```python
from build123d import *

# Parameters (mm, degrees)
F1_DEPTH = 3


with BuildPart() as f1:
    # F0 (on Top) → F1 (new body)
    with BuildSketch(Plane.XY):
        with BuildLine():
            Line((-2, 29.9332590942), (-2, 37.4466286867))
            ThreePointArc((-2, 37.4466286867), (-26.5165042945, 26.5165042945), (-37.4466286867, 2))
            Line((-37.4466286867, 2), (-29.9332590942, 2))
            ThreePointArc((-29.9332590942, 2), (-21.2132034356, 21.2132034356), (-2, 29.9332590942))
        make_face()
        with BuildLine():
            Line((-29.9332590942, -2), (-37.4466286867, -2))
            ThreePointArc((-37.4466286867, -2), (-26.5165042945, -26.5165042945), (-2, -37.4466286867))
            Line((-2, -37.4466286867), (-2, -29.9332590942))
            ThreePointArc((-2, -29.9332590942), (-21.2132034356, -21.2132034356), (-29.9332590942, -2))
        make_face()
        with BuildLine():
            Line((-14.8660687473, -2), (-27.4271763038, -2))
            ThreePointArc((-27.4271763038, -2), (-19.4454364826, -19.4454364826), (-2, -27.4271763038))
            Line((-2, -27.4271763038), (-2, -14.8660687473))
            ThreePointArc((-2, -14.8660687473), (-10.6066017178, -10.6066017178), (-14.8660687473, -2))
        make_face()
        with BuildLine():
            Line((-2, 14.8660687473), (-2, 27.4271763038))
            ThreePointArc((-2, 27.4271763038), (-19.4454364826, 19.4454364826), (-27.4271763038, 2))
            Line((-27.4271763038, 2), (-14.8660687473, 2))
            ThreePointArc((-14.8660687473, 2), (-10.6066017178, 10.6066017178), (-2, 14.8660687473))
        make_face()
        with BuildLine():
            ThreePointArc((27.4271763038, 2), (19.4454364826, 19.4454364826), (2, 27.4271763038))
            Line((2, 27.4271763038), (2, 14.8660687473))
            ThreePointArc((2, 14.8660687473), (10.6066017178, 10.6066017178), (14.8660687473, 2))
            Line((14.8660687473, 2), (27.4271763038, 2))
        make_face()
        with BuildLine():
            ThreePointArc((2, -27.4271763038), (19.4454364826, -19.4454364826), (27.4271763038, -2))
            Line((27.4271763038, -2), (14.8660687473, -2))
            ThreePointArc((14.8660687473, -2), (10.6066017178, -10.6066017178), (2, -14.8660687473))
            Line((2, -14.8660687473), (2, -27.4271763038))
        make_face()
        with BuildLine():
            ThreePointArc((2, -37.4466286867), (26.5165042945, -26.5165042945), (37.4466286867, -2))
            Line((37.4466286867, -2), (29.9332590942, -2))
            ThreePointArc((29.9332590942, -2), (21.2132034356, -21.2132034356), (2, -29.9332590942))
            Line((2, -29.9332590942), (2, -37.4466286867))
        make_face()
        with BuildLine():
            ThreePointArc((37.4466286867, 2), (26.5165042945, 26.5165042945), (2, 37.4466286867))
            Line((2, 37.4466286867), (2, 29.9332590942))
            ThreePointArc((2, 29.9332590942), (21.2132034356, 21.2132034356), (29.9332590942, 2))
            Line((29.9332590942, 2), (37.4466286867, 2))
        make_face()
        with BuildLine():
            Line((2, 14.8660687473), (2, 27.4271763038))
            ThreePointArc((2, 27.4271763038), (0, 27.5), (-2, 27.4271763038))
            Line((-2, 27.4271763038), (-2, 14.8660687473))
            ThreePointArc((-2, 14.8660687473), (0, 15), (2, 14.8660687473))
        make_face()
        with BuildLine():
            Line((2, 27.4271763038), (2, 29.9332590942))
            ThreePointArc((2, 29.9332590942), (0, 30), (-2, 29.9332590942))
            Line((-2, 29.9332590942), (-2, 27.4271763038))
            ThreePointArc((-2, 27.4271763038), (0, 27.5), (2, 27.4271763038))
        make_face()
        with BuildLine():
            Line((2, 29.9332590942), (2, 37.4466286867))
            Line((2, 37.4466286867), (-2, 37.4466286867))
            Line((-2, 37.4466286867), (-2, 29.9332590942))
            ThreePointArc((-2, 29.9332590942), (0, 30), (2, 29.9332590942))
        make_face()
        with BuildLine():
            Line((2, 12.3389626793), (2, 14.8660687473))
            ThreePointArc((2, 14.8660687473), (0, 15), (-2, 14.8660687473))
            Line((-2, 14.8660687473), (-2, 12.3389626793))
            ThreePointArc((-2, 12.3389626793), (0, 12.5), (2, 12.3389626793))
        make_face()
        with BuildLine():
            Line((2, 2.8722813233), (2, 12.3389626793))
            ThreePointArc((2, 12.3389626793), (0, 12.5), (-2, 12.3389626793))
            Line((-2, 12.3389626793), (-2, 2.8722813233))
            ThreePointArc((-2, 2.8722813233), (0, 3.5), (2, 2.8722813233))
        make_face()
        with BuildLine():
            Line((-2.8722813233, 2), (-12.3389626793, 2))
            ThreePointArc((-12.3389626793, 2), (-12.5, 0), (-12.3389626793, -2))
            Line((-12.3389626793, -2), (-2.8722813233, -2))
            ThreePointArc((-2.8722813233, -2), (-3.5, 0), (-2.8722813233, 2))
        make_face()
        with BuildLine():
            Line((-14.8660687473, 2), (-27.4271763038, 2))
            ThreePointArc((-27.4271763038, 2), (-27.5, 0), (-27.4271763038, -2))
            Line((-27.4271763038, -2), (-14.8660687473, -2))
            ThreePointArc((-14.8660687473, -2), (-15, 0), (-14.8660687473, 2))
        make_face()
        with BuildLine():
            Line((-12.3389626793, 2), (-14.8660687473, 2))
            ThreePointArc((-14.8660687473, 2), (-15, 0), (-14.8660687473, -2))
            Line((-14.8660687473, -2), (-12.3389626793, -2))
            ThreePointArc((-12.3389626793, -2), (-12.5, 0), (-12.3389626793, 2))
        make_face()
        with BuildLine():
            Line((-2, 2.8722813233), (-2, 12.3389626793))
            ThreePointArc((-2, 12.3389626793), (-8.8388347648, 8.8388347648), (-12.3389626793, 2))
            Line((-12.3389626793, 2), (-2.8722813233, 2))
            ThreePointArc((-2.8722813233, 2), (-2.4748737342, 2.4748737342), (-2, 2.8722813233))
        make_face()
        with BuildLine():
            Line((-2.8722813233, -2), (-12.3389626793, -2))
            ThreePointArc((-12.3389626793, -2), (-8.8388347648, -8.8388347648), (-2, -12.3389626793))
            Line((-2, -12.3389626793), (-2, -2.8722813233))
            ThreePointArc((-2, -2.8722813233), (-2.4748737342, -2.4748737342), (-2.8722813233, -2))
        make_face()
        with BuildLine():
            ThreePointArc((12.3389626793, 2), (8.8388347648, 8.8388347648), (2, 12.3389626793))
            Line((2, 12.3389626793), (2, 2.8722813233))
            ThreePointArc((2, 2.8722813233), (2.4748737342, 2.4748737342), (2.8722813233, 2))
            Line((2.8722813233, 2), (12.3389626793, 2))
        make_face()
        with BuildLine():
            ThreePointArc((2, -12.3389626793), (8.8388347648, -8.8388347648), (12.3389626793, -2))
            Line((12.3389626793, -2), (2.8722813233, -2))
            ThreePointArc((2.8722813233, -2), (2.4748737342, -2.4748737342), (2, -2.8722813233))
            Line((2, -2.8722813233), (2, -12.3389626793))
        make_face()
        with BuildLine():
            Line((-2, -2.8722813233), (-2, -12.3389626793))
            ThreePointArc((-2, -12.3389626793), (0, -12.5), (2, -12.3389626793))
            Line((2, -12.3389626793), (2, -2.8722813233))
            ThreePointArc((2, -2.8722813233), (0, -3.5), (-2, -2.8722813233))
        make_face()
        with BuildLine():
            Line((-2, -12.3389626793), (-2, -14.8660687473))
            ThreePointArc((-2, -14.8660687473), (0, -15), (2, -14.8660687473))
            Line((2, -14.8660687473), (2, -12.3389626793))
            ThreePointArc((2, -12.3389626793), (0, -12.5), (-2, -12.3389626793))
        make_face()
        with BuildLine():
            Line((-2, -14.8660687473), (-2, -27.4271763038))
            ThreePointArc((-2, -27.4271763038), (0, -27.5), (2, -27.4271763038))
            Line((2, -27.4271763038), (2, -14.8660687473))
            ThreePointArc((2, -14.8660687473), (0, -15), (-2, -14.8660687473))
        make_face()
        with BuildLine():
            Line((-2, -29.9332590942), (-2, -37.4466286867))
            Line((-2, -37.4466286867), (2, -37.4466286867))
            Line((2, -37.4466286867), (2, -29.9332590942))
            ThreePointArc((2, -29.9332590942), (0, -30), (-2, -29.9332590942))
        make_face()
        with BuildLine():
            Line((-2, -27.4271763038), (-2, -29.9332590942))
            ThreePointArc((-2, -29.9332590942), (0, -30), (2, -29.9332590942))
            Line((2, -29.9332590942), (2, -27.4271763038))
            ThreePointArc((2, -27.4271763038), (0, -27.5), (-2, -27.4271763038))
        make_face()
        with BuildLine():
            ThreePointArc((15, 0), (14.9664797332, 1.0022396895), (14.8660687473, 2))
            Line((14.8660687473, 2), (12.3389626793, 2))
            ThreePointArc((12.3389626793, 2), (12.4596756276, 1.0032363902), (12.5, 0))
            ThreePointArc((12.5, 0), (12.4596756276, -1.0032363902), (12.3389626793, -2))
            Line((12.3389626793, -2), (14.8660687473, -2))
            ThreePointArc((14.8660687473, -2), (14.9664797332, -1.0022396895), (15, 0))
        make_face()
        with BuildLine():
            ThreePointArc((12.5, 0), (12.4596756276, 1.0032363902), (12.3389626793, 2))
            Line((12.3389626793, 2), (2.8722813233, 2))
            ThreePointArc((2.8722813233, 2), (3.3393850206, 1.0480971731), (3.5, 0))
            ThreePointArc((3.5, 0), (3.3393850206, -1.0480971731), (2.8722813233, -2))
            Line((2.8722813233, -2), (12.3389626793, -2))
            ThreePointArc((12.3389626793, -2), (12.4596756276, -1.0032363902), (12.5, 0))
        make_face()
        with BuildLine():
            ThreePointArc((27.5, 0), (27.4817880455, 1.0006626918), (27.4271763038, 2))
            Line((27.4271763038, 2), (14.8660687473, 2))
            ThreePointArc((14.8660687473, 2), (14.9664797332, 1.0022396895), (15, 0))
            ThreePointArc((15, 0), (14.9664797332, -1.0022396895), (14.8660687473, -2))
            Line((14.8660687473, -2), (27.4271763038, -2))
            ThreePointArc((27.4271763038, -2), (27.4817880455, -1.0006626918), (27.5, 0))
        make_face()
        with BuildLine():
            ThreePointArc((37.5, 0), (37.4866547971, 1.0003559988), (37.4466286867, 2))
            Line((37.4466286867, 2), (29.9332590942, 2))
            ThreePointArc((29.9332590942, 2), (29.983310131, 1.0005566386), (30, 0))
            ThreePointArc((30, 0), (29.983310131, -1.0005566386), (29.9332590942, -2))
            Line((29.9332590942, -2), (37.4466286867, -2))
            ThreePointArc((37.4466286867, -2), (37.4866547971, -1.0003559988), (37.5, 0))
        make_face()
        with BuildLine():
            Line((-29.9332590942, 2), (-37.4466286867, 2))
            ThreePointArc((-37.4466286867, 2), (-37.5, 0), (-37.4466286867, -2))
            Line((-37.4466286867, -2), (-29.9332590942, -2))
            ThreePointArc((-29.9332590942, -2), (-30, 0), (-29.9332590942, 2))
        make_face()
    extrude(amount=F1_DEPTH)


solid = f1.part
```
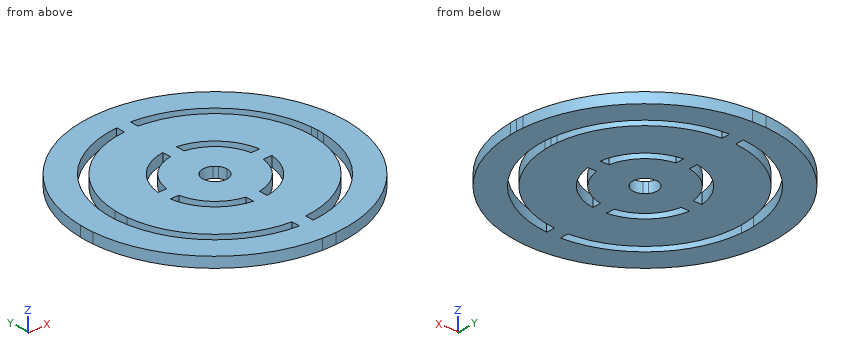
Part model, mm, in its own coordinate system. Round coordinates to 2 decimals unless told otherwise and drop trailing zeros. Write each loop counter-clockwise with the first axis right and the second up, starting at its lowest first coordinate (ties: lowest second). Pieces come first, ordered by that corner, then holes. Notation, with made-up numbers: M -27.5,-32.75 L -14.5,-32.75 A4 cw -14.5,-26.75 Z; hole C -21,85 d2. An arc over 180 degrees is marked long. Answer as CSV lines item,"result". Start each with the question number.
1) Drill centre lines: L1, parallel to X at y = -15, z = 0.6; L2, parallel to X at y = -13.5, z = 1.3; L3, parallel to X at y = 10, z = 1.55. Where is each one in solid material? Low to high.
2) Drop flat-ended pins along their axis: pin 1 (0.8 mm diameter, centred on y = 13.5, z = 1.5, fed in from -X); pin 2 (1.3 mm diameter, centred on x = -13.5, z = 1.5, fed in from -Y); pin 3 (1.3 mm diameter, centred on y = -13.5, z = 1.5, fed in from +X). Give the stop position or say it passes through.
3) Band-saw the part on D-D (z = 1). Count the separate pieces of the cut face and the enclosed holes in it, then the cut area to 3 significant figures.
4) Band-saw the part on B-B (y = 20.5). List the corners of the cut face in (x, z).
5) Band-saw the part on A-A (x = 0). List the corners of the cut face in (y, z).
6) Band-saw the part on C-C (y = 7). List the corners of the cut face in (x, z), then the cut area to 3 significant figures.
Worked out:
1,L1,"-34.37 to -25.98, -23.05 to 23.05, 25.98 to 34.37"
1,L2,"-34.99 to -26.79, -23.96 to -6.54, -2 to 2, 6.54 to 23.96, 26.79 to 34.99"
1,L3,"-36.14 to -28.28, -25.62 to -11.18, -7.5 to 7.5, 11.18 to 25.62, 28.28 to 36.14"
2,pin 1,"x = -35.14"
2,pin 2,"y = -35.23"
2,pin 3,"x = 35.23"
3,separate pieces,"1"
3,enclosed holes,"7"
3,area,"3,770 mm²"
4,outline,"M -31.4,0 L -21.9,0 L -21.9,3 L -31.4,3 Z; M -18.33,0 L 18.33,0 L 18.33,3 L -18.33,3 Z; M 21.9,0 L 31.4,0 L 31.4,3 L 21.9,3 Z"
5,outline,"M -37.45,0 L -3.5,0 L -3.5,3 L -37.45,3 Z; M 3.5,0 L 37.45,0 L 37.45,3 L 3.5,3 Z"
6,outline,"M -36.84,0 L -29.17,0 L -29.17,3 L -36.84,3 Z; M -26.59,0 L -13.27,0 L -13.27,3 L -26.59,3 Z; M -10.36,0 L 10.36,0 L 10.36,3 L -10.36,3 Z; M 13.27,0 L 26.59,0 L 26.59,3 L 13.27,3 Z; M 29.17,0 L 36.84,0 L 36.84,3 L 29.17,3 Z"
6,area,"188 mm²"
